Geometry check sheet. Reference: the model listing, model coordinates, mm. A direction names the side the tool comes from. Round coordinates to 2 decimals unless told otherwise and drop trailing zeros. Write each loop counter-clockwise with the first axis right and the second up, starting at its lowest first coordinate (ties: lowest second). Pieces come first, ordered by that corner, then holes. Notation, with made-up numbers: M -39.5,88 L -31.5,88 A17 cw -31.5,114 Z; hole C -18.5,24.25 d10. An arc over 180 degrees is marked long. One line per item, written item: value. Start each with the question number.
1. Section check D-D (x = -59.5). Record the boundary of the cut face in (y, z).
2. Scan lines: probe 1 along Y at (x, z) = (-59, 32.5); probe 2 along Z at (x, y) = (-63.5, 55.25); probe 3 along Y at (x, z) = (-62.75, 35). Record each from-to range of solid material in increasing order. Write a range as [from, to].
3. Depth check by flat-ended pin: P1, Ø3, axis at y = 50.5, z = 32.5, coming from the -X side. Enter the tip coordinate at first touch or a pass-through.
4. Section check C-C (z = 34.5). Record the boundary of the cut face in (x, y), and give its area (3 significant figures).
5. Release check for a two-part mould opening along Y. For faces 1 (the flat face through (-60, 57.4, 32)), 2 (the flat face through (-62, 48, 32)), 3 (the flat face through (-61, 59, 33)) record: pulls with the +Y half, pulls with the -Y half, needs draft (parallel to the pull), parting line crosses it, or undercut.
6. Section check A-A (x = -63.5). Record the boundary of the cut face in (y, z), and give its area (3 significant figures).
7. Section check B-B (z = 29.75). Record the boundary of the cut face in (x, y).
8. Access from +Z, -Z, +X, -X, +Y, -Y to the whole of each face (thin tool, end or side, straight path). Record for faces 4 (the flat face through (-64, 51.4, 35)), 5 (the flat face through (-62, 58, 32)).
from build123d import *

# Parameters (mm, degrees)
PAD040_DEPTH            = 1.2
PAD041_DEPTH            = 1.6
LINEARPATTERN003_COUNT  = 2
LINEARPATTERN003_PITCH  = 10.4
FILLET009_R             = 1
FILLET010_R             = 1
FILLET011_R             = 1
BODY013_PLACEMENT_ANGLE = 180


with BuildPart() as part:
    # Sketch072 → Pad040 (new body)
    with BuildSketch(Plane.XY):
        with BuildLine():
            Line((-4, 6), (4, 6))
            Line((4, 6), (4, 1.6))
            Line((1, 1.6), (4, 1.6))
            ThreePointArc((1, 1.6), (-0.6, 0), (1, -1.6))
            Line((4, -1.6), (1, -1.6))
            Line((4, -1.6), (4, -6))
            Line((4, -6), (-4, -6))
            Line((-4, -6), (-4, 6))
        make_face()
    extrude(amount=PAD040_DEPTH)

    # Sketch073 (on DatumPlane) → Pad041 (join)
    with BuildSketch(Plane.XZ.offset(6)):
        Polygon((-4, 0), (-4, -6), (-2, -6), (-2, -4.4), (2, 0), align=None)
    pad041 = extrude(amount=-PAD041_DEPTH)

    # LinearPattern003: Pad041 ×2
    with Locations(*[(0, i * LINEARPATTERN003_PITCH, 0) for i in range(1, LINEARPATTERN003_COUNT)]):
        add(pad041)

    # Fillet009
    fillet009_edges = [part.edges().sort_by_distance(p)[0] for p in [
        (-2, -5.2, -6),
        (-2, 5.2, -6),
    ]]
    fillet(fillet009_edges, radius=FILLET009_R)

    # Fillet010
    fillet010_edges = [part.edges().sort_by_distance(p)[0] for p in [
        (-2, -5.2, -4.4),
        (-2, 5.2, -4.4),
    ]]
    fillet(fillet010_edges, radius=FILLET010_R)

    # Fillet011
    fillet011_edges = [part.edges().sort_by_distance(p)[0] for p in [
        (4, -6, 0.6),
        (4, -1.6, 0.6),
        (4, 1.6, 0.6),
        (4, 6, 0.6),
    ]]
    fillet(fillet011_edges, radius=FILLET011_R)


with BuildPart() as part_1:
    # Body013 placement: moved
    add(part.part.moved(Location((-62, 53, 34.2))).rotate(Axis((-62, 53, 34.2), (0, 0, 1)), BODY013_PLACEMENT_ANGLE))


solid = part_1.part
Result sheet:
1. outline: M 47,28.33 L 48.6,28.33 L 48.6,34.2 L 57.4,34.2 L 57.4,28.33 L 59,28.33 L 59,35.4 L 47,35.4 Z
2. probe 1: y = [47, 48.6], [57.4, 59]
2. probe 2: z = [34.2, 35.4]
2. probe 3: y = [47, 51.42], [54.58, 59]
3. P1: passes through
4. outline: M -66,48 A1 ccw -65,47 L -58,47 L -58,59 L -65,59 A1 ccw -66,58 L -66,55.6 A1 ccw -65,54.6 L -63,54.6 A1.6 cw -63,51.4 L -65,51.4 A1 ccw -66,50.4 Z
4. area: 81.5 mm2
5. face 1: undercut
5. face 2: needs draft
5. face 3: pulls with the +Y half
6. outline: M 47,33.65 L 48.6,33.65 L 48.6,34.2 L 51.4,34.2 L 51.4,35.4 L 47,35.4 Z; M 54.6,34.2 L 57.4,34.2 L 57.4,33.65 L 59,33.65 L 59,35.4 L 54.6,35.4 Z
6. area: 12.3 mm2
7. outline: M -60.06,47 L -58,47 L -58,48.6 L -60.06,48.6 Z; M -60.06,57.4 L -58,57.4 L -58,59 L -60.06,59 Z
8. face 4: +Z, -Z, -X
8. face 5: -Z, -X, +Y, -Y
